Verification items for the finished model (mm, model axes). Face numbers are marked on the shaded views. A direction names the side the tool comes from. Round coordinates to 2 decimals unless told otherwise and drop trailing zeros. Write each loop counter-clockwise with the first axis right and the second up, starting at its lowest first coordinate (ties: lowest second). Pieces come first, ordered by that corner, then holes. Notation, with made-up numbers: (45, -34.5) -> (67, -34.5) arc R26 ccw to (67, -17.5) -> close; hole circle Ø7 at (63.25, 78). An arc over 180 degrees is marked (long way). Answer as a JSON object with one key per item and string values. Group by question number.
(1) Draft check along X on the marked faces 3, 4 and 5. Enter one of: released by +X, released by -X, zero draft, split by the parting line, or undercut.
(2) Sectioned sample at A-A on y = 0. Record the cut outline in (x, z).
(3) Sectioned sample at D-D on x = -24. Count the separate pieces of the cut face and the enclosed holes in it, and give its area (3 significant figures).
(4) Sectioned sample at C-C on x = 0. Record the cut outline in (y, z).
(5) Sectioned sample at B-B on z = 7.5. Record the cut outline in (x, y).
(6) Set-up check for the marked faces 1 and 2: record each of +Z, -Z, +X, -X, +Y, -Y from which the full face is reachable in a straight line by a thin tool's end or side.
(7) Gauge pin test, flat ends, axial feed: pin 1 Ø4 at (y, z) = (-10.5, 1.5) entering from -X; pin 2 Ø2.5 at (x, y) = (-24.75, -24.75) entering from -Z; pin 3 Ø4 at (x, z) = (7, 7) entering from +Y; pin 4 Ø1 at (x, z) = (-2, 5) entering from -Y. Record the tip position at first contact, or that the pin passes through.
(8) Scan lines: L1, parallel to X at y = -34.5, z = 6; L2, parallel to Y at x = 8, z = 7.5; L3, parallel to X at y = 20, z = 2.25. Record each from-to range of solid material in increasing order. Write a range as from..to.
```python
from build123d import *

# Parameters (mm, degrees)
SKETCH_1_R               = 40
SKETCH_1_R_2             = 30.5
EXTRUDE_1_DEPTH          = 12
SKETCH_2_R               = 1.7
CUT_EXTRUDE_1_DEPTH      = 12
FILLET_1_R               = 2
FILLET_2_R               = 2
CUT_EXTRUDE_2_DEPTH      = 10
CUT_EXTRUDE_2_DEPTH_BACK = 58.827329248
SKETCH_3_W               = 10
SKETCH_3_H               = 17.135936663


with BuildPart() as part:
    # 草图1 → 凸台-拉伸1 (new body)
    with BuildSketch(Plane.XY):
        Circle(SKETCH_1_R)
        Circle(SKETCH_1_R_2, mode=Mode.SUBTRACT)
    extrude(amount=EXTRUDE_1_DEPTH)

    # 草图2 → 切除-拉伸1 (cut)
    with BuildSketch(Plane.XY.offset(12)):
        with Locations((24.748737342, 24.748737342)):
            Circle(SKETCH_2_R)
        with Locations((24.748737342, -24.748737342)):
            Circle(SKETCH_2_R)
        with Locations((-24.748737342, -24.748737342)):
            Circle(SKETCH_2_R)
        with Locations((-24.748737342, 24.748737342)):
            Circle(SKETCH_2_R)
    extrude(amount=-CUT_EXTRUDE_1_DEPTH, mode=Mode.SUBTRACT)

    # 圆角1
    fillet_1_edges = [part.edges().sort_by_distance(p)[0] for p in [
        (-30.5, 0, 12),
    ]]
    fillet(fillet_1_edges, radius=FILLET_1_R)

    # 圆角2
    fillet_2_edges = [part.edges().sort_by_distance(p)[0] for p in [
        (-40, 0, 12),
    ]]
    fillet(fillet_2_edges, radius=FILLET_2_R)

    # 草图3 → 切除-拉伸2 (cut, two sides: drawn at the far end of the back side and taken through both)
    with BuildSketch(Plane(origin=(0, 0, 0), x_dir=(1, 0, 0), z_dir=(0, 1, 0)).offset(-CUT_EXTRUDE_2_DEPTH_BACK)):
        with Locations((0, -8.567968332)):
            Rectangle(SKETCH_3_W, SKETCH_3_H)
    extrude(amount=CUT_EXTRUDE_2_DEPTH + CUT_EXTRUDE_2_DEPTH_BACK, mode=Mode.SUBTRACT)


solid = part.part
```
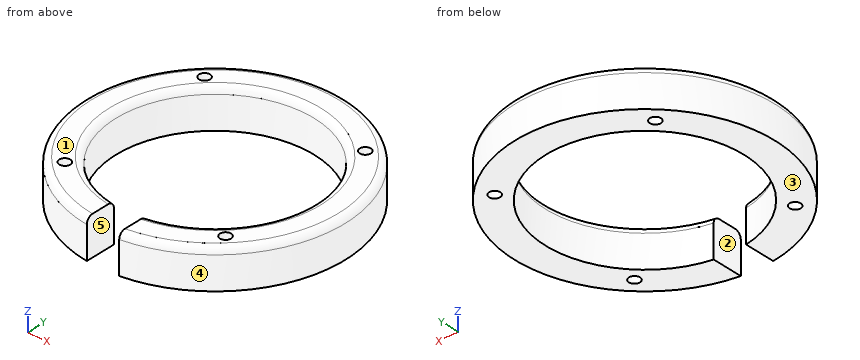
Computed values:
{
 "1": {"face 3": "zero draft", "face 4": "split by the parting line", "face 5": "undercut"},
 "2": {"outline": "(-40, 0) -> (-30.5, 0) -> (-30.5, 10) arc R2 ccw to (-32.5, 12) -> (-38, 12) arc R2 ccw to (-40, 10) -> close; (30.5, 0) -> (40, 0) -> (40, 10) arc R2 ccw to (38, 12) -> (32.5, 12) arc R2 ccw to (30.5, 10) -> close"},
 "3": {"separate pieces": "4", "enclosed holes": "0", "area": "238 mm2"},
 "4": {"outline": "(30.5, 0) -> (40, 0) -> (40, 10) arc R2 ccw to (38, 12) -> (32.5, 12) arc R2 ccw to (30.5, 10) -> close"},
 "5": {"outline": "(-5, -39.69) -> (-5, -30.09) arc R30.5 cw (long way) to (5, -30.09) -> (5, -39.69) arc R40 ccw (long way) to start; hole circle Ø3.4 at (-24.75, -24.75); hole circle Ø3.4 at (-24.75, 24.75); hole circle Ø3.4 at (24.75, -24.75); hole circle Ø3.4 at (24.75, 24.75)"},
 "6": {"face 1": "+Z, +X, -X, +Y, -Y", "face 2": "+Z, -Z, -Y"},
 "7": {"pin 1": "x = -39.09", "pin 2": "through", "pin 3": "y = 39.69", "pin 4": "y = 30.4"},
 "8": {"L1": "-20.24..-5, 5..20.24", "L2": "-39.19..-29.43, 29.43..39.19", "L3": "-34.64..-23.03, 23.03..34.64"}
}
